Autodesk Inventor part; units mm, degrees
ref_plane "YZ Plane" through (0, 0, 0) normal (1, 0, 0) x (0, 1, 0)
ref_plane "XZ Plane" through (0, 0, 0) normal (0, 1, 0) x (-1, 0, 0)
ref_plane "XY Plane" through (0, 0, 0) normal (0, 0, 1) x (1, 0, 0)
sketch "Sketch1" plane through (0, 0, 0) normal (0, 1, 0) x (-1, 0, 0)
  circle A0 centre (0, 0) radius 45
  circle A1 centre (0, 0) radius 35
  dimension "d0" = 10
  dimension "d1" = 70
extrude "Extrusion1" add sketch "Sketch1" along normal blind 2
sketch "Sketch2" plane through (0, 2, 0) normal (0, 1, 0) x (1, 0, 0)
  circle A0 centre (0, 40) radius 1.5
  line L0 (0, 0) -> (0, 64.6181) construction
  circle A1 centre (-38.0423, 12.3607) radius 1.5
  line L1 (0, 0) -> (-61.4554, 19.9681) construction
  circle A2 centre (-23.5114, -32.3607) radius 1.5
  line L2 (0, 0) -> (-37.9816, -52.2771) construction
  circle A3 centre (23.5114, -32.3607) radius 1.5
  line L3 (0, 0) -> (37.9816, -52.2771) construction
  circle A4 centre (38.0423, 12.3607) radius 1.5
  line L4 (0, 0) -> (61.4554, 19.9681) construction
  dimension "d4" = 3
  dimension "d5" = 40
  dimension "d8" = 360
extrude "Extrusion2" cut sketch "Sketch2" against normal blind 3
properties part number "HeatingElementHolder01"
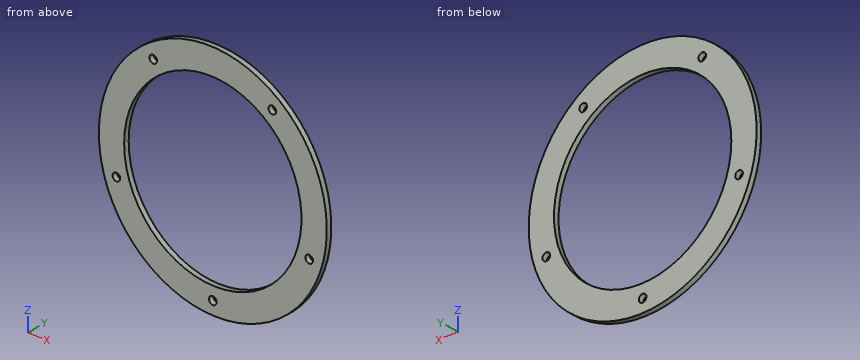
The listing builds one solid part. Answer for the finished solid, in the listing's coordinates (mm). Round coordinates to 2 decimals unless told otherwise and drop trailing zeros. Loops run counter-clockwise (first coordinate to the right, second up) from the corner with the lowest first, then second, coordinate; pieces in that order, holes last. Notation, with made-up numbers: M 25.5,1.5 L 42.5,1.5 A24 cw 42.5,28.5 Z; hole C 54.25,-5 d6. An arc over 180 degrees is marked long. Write each question's results on one line, items separated by ' | '. Start each with the question number.
1) Find section A-A on x = 0. Write down the section's boundary in (y, z), plus the area to 3 significant figures.
2) Find section D-D on y = 0.75. Write down the section's boundary in (x, z).
3) This flat-tipped pin is pushed along its axis until it touches: pin 1 (1 mm diameter, centred on y = 2, z = -6.5, fed in from +X). Where does it stop, or does it pass through?
4) Straight lines are drawn through the part: probe 1 along Z at (x, y) = (0, 0.5); probe 2 along Z at (x, y) = (23, 0.45); probe 3 along Z at (x, y) = (-31, 1.15). For each, find the intervals that lie inside material, in ascending order.
5) Find section C-C on x = 16.5. Write down the section's boundary in (y, z), plus the area to 3 significant figures.
6) Find section B-B on z = 0. Write down the section's boundary in (x, y), plus the area to 3 significant figures.
Final values:
1) outline: M 0,-45 L 2,-45 L 2,-41.5 L 0,-41.5 Z; M 0,-38.5 L 2,-38.5 L 2,-35 L 0,-35 Z; M 0,35 L 2,35 L 2,45 L 0,45 Z | area: 34.0 mm²
2) outline: C 0,0 d90; hole C -38.04,-12.36 d3; hole C 0,0 d70; hole C -23.51,32.36 d3; hole C 0,-40 d3; hole C 23.51,32.36 d3; hole C 38.04,-12.36 d3
3) pin 1: x = 44.6
4) probe 1: -45 to -41.5, -38.5 to -35, 35 to 45 | probe 2: -38.68 to -26.38, 26.38 to 30.95, 33.77 to 38.68 | probe 3: -32.62 to -16.25, 16.25 to 32.62
5) outline: M 0,-41.87 L 2,-41.87 L 2,-30.87 L 0,-30.87 Z; M 0,30.87 L 2,30.87 L 2,41.87 L 0,41.87 Z | area: 44.0 mm²
6) outline: M -45,0 L -35,0 L -35,2 L -45,2 Z; M 35,0 L 45,0 L 45,2 L 35,2 Z | area: 40.0 mm²
